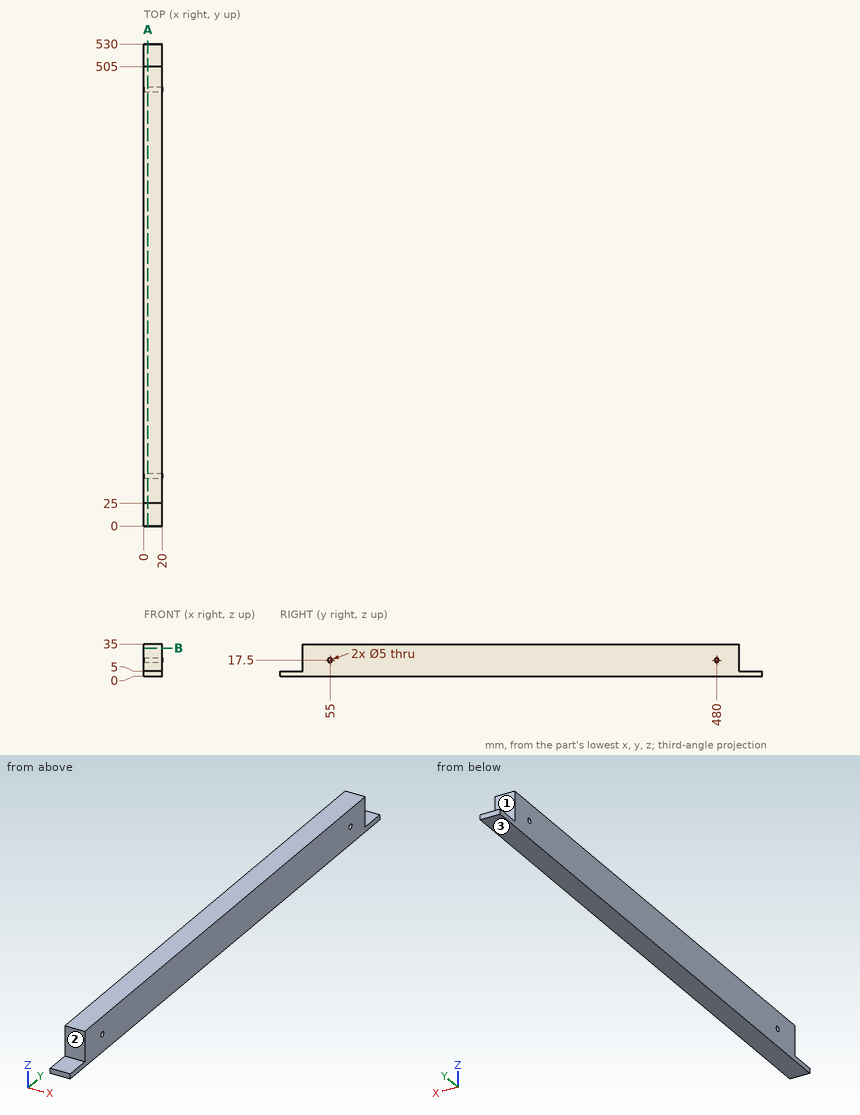
Answer from the drawing. Dimensions are ordinates in mm from the lowest x, y and z of the part. A direction names the side the tool comes from. Give positions to 0.01 mm unless a question says otherwise; leave off trailing zeros. Loops run counter-clockwise (first coordinate to the right, second up) from the corner with the lowest first, then second, coordinate; pieces in that order, holes last. Notation, with made-up numbers: M -29.75,1.5 L 27.25,1.5 A16 ccw 27.25,5.5 Z; hole C 49,14 d1. An arc over 180 degrees is marked long. One line per item, written item: value.
Q1. For the marked faces 1, 2 and 3, determine the directions among +Z, -Z, +X, -X, +Y, -Y from which every point of the face is accessible in a straight line to the end or side of a thin tool.
Working result:
face 1: +Z, +X, -X, +Y
face 2: +Z, +X, -X, -Y
face 3: -Z, +X, -X, +Y, -Y
Q2. Find the intervals of material crossed by line 1 (Z direction, x = 9.75, y = 480); line 2 (Y direction, x = 6.75, z = 25.5); line 3 (Z direction, x = 18.5, y = 55.5), in increasing order. Write a range as from..to.
Working result:
line 1: z = 0..15, 20..35
line 2: y = 25..505
line 3: z = 0..15.05, 19.95..35
Q3. A cutting plane is placed at B-B on z = 30.5. Determine the outline of the cut face in (x, y), then the cut area to 3 significant figures.
Working result:
outline: M 0,25 L 20,25 L 20,505 L 0,505 Z
area: 9,600 mm^2
Q4. Flat-ended cylindrical pins translate along their axes: P1, Ø10, axis at x = 10, y = 12, coming from the +Z side; P2, Ø4, axis at x = 12, z = 14, coming from the +Y side; P3, Ø10, axis at x = 8.5, z = 17.5, coming from the -Y side. Find the tip coordinate at first contact, or state that the pin passes through.
Working result:
P1: stops at z = 5
P2: stops at y = 505
P3: stops at y = 25
Q5. A cutting plane is placed at A-A on x = 4.5. Determine the outline of the cut face in (y, z).
Working result:
outline: M 0,0 L 530,0 L 530,5 L 505,5 L 505,35 L 25,35 L 25,5 L 0,5 Z; hole C 55,17.5 d5; hole C 480,17.5 d5
